Read the model definition and answer for the solid it produces. Units are mm, in the model's axes. A direction names the side the tool comes from. Give positions to 0.01 mm unless a question says otherwise; leave off trailing zeros. Order: outer loops, then holes, each group sorted by start corner. A loop starts at its lowest first (then second) coordinate and runs counter-clockwise, first axis right, second up. Notation, with made-up numbers: (19.25, 41.25) - (78.25, 41.25) arc R20 cw to (78.25, 49.25) - close; hole circle Ø10 at (24, -1.5). An arc over 180 degrees is marked (long way). Use a Markdown table: item, result. Add a question column.
1. Flat-ended cylindrical pins translate along their axes: P1, Ø10, axis at y = 5.5, z = 41.5, coming from the +X side; P2, Ø6, axis at y = 28, z = 19.5, coming from the -X side; P3, Ø2.5, axis at x = -61.5, z = 42.5, coming from the +Y side. Find the tip coordinate at first contact, or state that the pin passes through.
2. Which of the six approach directions +Z, -Z, +X, -X, +Y, -Y give full straight-line access (tool end or side, diameter ignored) to faces 4 (the flat face through (-49, -2, 30)), 5 (the flat face through (-35, 30, 32)), 6 (the flat face through (-62, 21, 16)), 7 (the flat face through (-37.5, 12, 38)), 8 (the flat face through (-68, -2, 30))?
3. A cutting plane is placed at D-D on y = 1. Determine the outline of the cut face in (x, z), and give its area (3 significant figures).
4. A cutting plane is placed at B-B on z = 46.5. Determine the outline of the cut face in (x, y).
5. Consider L1, parallel to X at y = 20, z = 38; L2, parallel to X at y = 37, z = 2; L3, parallel to Z at x = -35.5, y = 2.5. Determine where each line is inside the solid, lowest interval first.
6. A cutting plane is placed at C-C on x = -52.5. Determine the outline of the cut face in (y, z).
7. A cutting plane is placed at A-A on y = 37.5. Determine the outline of the cut face in (x, z), and give its area (3 significant figures).
8. For a pull along Z with two mould halves and no side action, classify faces 1 (the flat face through (-35, 10, 26)), 2 (the flat face through (-3, -2, 30)), 3 (the flat face through (-32.5, 12, 38)) as released by +Z, released by -Z, zero draft, split by the parting line, or undercut.
```python
from build123d import *

# Parameters (mm, degrees)
SKETCH1_W           = 70
SKETCH1_H           = 50
BOSS_EXTRUDE1_DEPTH = 5
SKETCH2_W           = 5
SKETCH2_H           = 30
BOSS_EXTRUDE2_DEPTH = 25
SKETCH3_W           = 21
SKETCH3_H           = 21
CUT_EXTRUDE1_DEPTH  = 5
SKETCH4_W           = 21
SKETCH4_H           = 21
CUT_EXTRUDE2_DEPTH  = 5
SKETCH5_W           = 21
SKETCH5_H           = 21
CUT_EXTRUDE3_DEPTH  = 5
SKETCH6_W           = 70
SKETCH6_H           = 30
BOSS_EXTRUDE3_DEPTH = 5
SKETCH7_W           = 5
SKETCH7_H           = 35
BOSS_EXTRUDE4_DEPTH = 35
SKETCH8_R           = 6.5
CUT_EXTRUDE4_DEPTH  = 5
SKETCH9_W           = 5
SKETCH9_H           = 35
CUT_EXTRUDE5_DEPTH  = 5
SKETCH10_W          = 20
SKETCH10_H          = 5
CUT_EXTRUDE6_DEPTH  = 5
SKETCH11_W          = 20
SKETCH11_H          = 5
CUT_EXTRUDE7_DEPTH  = 5


with BuildPart() as part:
    # Sketch1 → Boss-Extrude1 (new body)
    with BuildSketch(Plane.XY):
        with Locations((-35, 25)):
            Rectangle(SKETCH1_W, SKETCH1_H)
    extrude(amount=BOSS_EXTRUDE1_DEPTH)

    # Sketch2 → Boss-Extrude2 (add)
    with BuildSketch(Plane.XY.offset(5)):
        with Locations((-62.5, 15)):
            Rectangle(SKETCH2_W, SKETCH2_H)
        with Locations((-35, 15)):
            Rectangle(SKETCH2_W, SKETCH2_H)
        with Locations((-7.5, 15)):
            Rectangle(SKETCH2_W, SKETCH2_H)
    extrude(amount=BOSS_EXTRUDE2_DEPTH)

    # Sketch3 → Cut-Extrude1 (cut)
    with BuildSketch(Plane(origin=(-5, 0, 0), x_dir=(0, 0, -1), z_dir=(1, 0, 0))):
        with Locations((-15.5, 10.5)):
            Rectangle(SKETCH3_W, SKETCH3_H)
    extrude(amount=-CUT_EXTRUDE1_DEPTH, mode=Mode.SUBTRACT)

    # Sketch4 → Cut-Extrude2 (cut)
    with BuildSketch(Plane(origin=(-32.5, 0, 0), x_dir=(0, 0, -1), z_dir=(1, 0, 0))):
        with Locations((-15.5, 10.5)):
            Rectangle(SKETCH4_W, SKETCH4_H)
    extrude(amount=-CUT_EXTRUDE2_DEPTH, mode=Mode.SUBTRACT)

    # Sketch5 → Cut-Extrude3 (cut)
    with BuildSketch(Plane(origin=(-60, 0, 0), x_dir=(0, 0, -1), z_dir=(1, 0, 0))):
        with Locations((-15.5, 10.5)):
            Rectangle(SKETCH5_W, SKETCH5_H)
    extrude(amount=-CUT_EXTRUDE3_DEPTH, mode=Mode.SUBTRACT)

    # Sketch6 → Boss-Extrude3 (add)
    with BuildSketch(Plane.XZ):
        with Locations((-35, 15)):
            Rectangle(SKETCH6_W, SKETCH6_H)
    extrude(amount=BOSS_EXTRUDE3_DEPTH)

    # Sketch7 → Boss-Extrude4 (add)
    with BuildSketch(Plane.XY.offset(30)):
        with Locations((-35, 12.5)):
            Rectangle(SKETCH7_W, SKETCH7_H)
        with Locations((-7.5, 12.5)):
            Rectangle(SKETCH7_W, SKETCH7_H)
        with Locations((-62.5, 12.5)):
            Rectangle(SKETCH7_W, SKETCH7_H)
    extrude(amount=BOSS_EXTRUDE4_DEPTH)

    # Sketch8 → Cut-Extrude4 (cut)
    with BuildSketch(Plane(origin=(0, 0, 0), x_dir=(-1, 0, 0), z_dir=(0, 0, -1))):
        with Locations((17.5, 37.5)):
            Circle(SKETCH8_R)
        with Locations((52.5, 37.5)):
            Circle(SKETCH8_R)
    extrude(amount=-CUT_EXTRUDE4_DEPTH, mode=Mode.SUBTRACT)

    # Sketch9 → Cut-Extrude5 (cut)
    with BuildSketch(Plane.XY.offset(65)):
        with Locations((-35, 12.5)):
            Rectangle(SKETCH9_W, SKETCH9_H)
    extrude(amount=-CUT_EXTRUDE5_DEPTH, mode=Mode.SUBTRACT)

    # Sketch10 → Cut-Extrude6 (cut)
    with BuildSketch(Plane(origin=(-5, 0, 0), x_dir=(0, 0, -1), z_dir=(1, 0, 0))):
        with Locations((-45, 2.5)):
            Rectangle(SKETCH10_W, SKETCH10_H)
    extrude(amount=-CUT_EXTRUDE6_DEPTH, mode=Mode.SUBTRACT)

    # Sketch11 → Cut-Extrude7 (cut)
    with BuildSketch(Plane.ZY.offset(65)):
        with Locations((45, 2.5)):
            Rectangle(SKETCH11_W, SKETCH11_H)
    extrude(amount=-CUT_EXTRUDE7_DEPTH, mode=Mode.SUBTRACT)


solid = part.part
```
Output values:
| question | item | result |
|---|---|---|
| 1 | P1 | x = -5 |
| 1 | P2 | x = -65 |
| 1 | P3 | y = 30 |
| 2 | face 4 | +Z, +Y, -Y |
| 2 | face 5 | +Z, +X, -X, +Y |
| 2 | face 6 | +X, -X |
| 2 | face 7 | +Z, +Y |
| 2 | face 8 | +Z, -X, +Y, -Y |
| 3 | outline | (-70, 0) - (0, 0) - (0, 5) - (-70, 5) - close; (-65, 26) - (-60, 26) - (-60, 35) - (-65, 35) - close; (-65, 55) - (-60, 55) - (-60, 65) - (-65, 65) - close; (-37.5, 26) - (-32.5, 26) - (-32.5, 60) - (-37.5, 60) - close; (-10, 26) - (-5, 26) - (-5, 35) - (-10, 35) - close; (-10, 55) - (-5, 55) - (-5, 65) - (-10, 65) - close |
| 3 | area | 710 mm² |
| 4 | outline | (-65, -5) - (-60, -5) - (-60, 0) - (-65, 0) - close; (-65, 5) - (-60, 5) - (-60, 30) - (-65, 30) - close; (-37.5, -5) - (-32.5, -5) - (-32.5, 30) - (-37.5, 30) - close; (-10, -5) - (-5, -5) - (-5, 0) - (-10, 0) - close; (-10, 5) - (-5, 5) - (-5, 30) - (-10, 30) - close |
| 5 | L1 | -65 to -60, -37.5 to -32.5, -10 to -5 |
| 5 | L2 | -70 to -58.98, -46.02 to -23.98, -11.02 to 0 |
| 5 | L3 | 0 to 5, 26 to 60 |
| 6 | outline | (-5, 0) - (31, 0) - (31, 5) - (0, 5) - (0, 30) - (-5, 30) - close; (44, 0) - (50, 0) - (50, 5) - (44, 5) - close |
| 7 | outline | (-70, 0) - (-59, 0) - (-59, 5) - (-70, 5) - close; (-46, 0) - (-24, 0) - (-24, 5) - (-46, 5) - close; (-11, 0) - (0, 0) - (0, 5) - (-11, 5) - close |
| 7 | area | 220 mm² |
| 8 | face 1 | undercut |
| 8 | face 2 | released by +Z |
| 8 | face 3 | zero draft |
